For this review, take the finished solid that the model builds, in its own axes (mm). A direction names the side the tool comes from. Give positions to 0.01 mm unless a question says otherwise; leave off trailing zeros. Loops run counter-clockwise (first coordinate to the right, second up) from the corner with the lowest first, then second, coordinate; pieces in that order, holes last. Notation, with made-up numbers: M -38,-15.5 L -17,-15.5 A25 cw -17,16.5 Z; hole C 34.5,43.5 d9. An arc over 180 degrees is marked long. Use CSV: the item, a comma, the result in double quotes. Start each with the question number.
1. Insertion check: P1, Ø5, axis at x = 10.5, z = 10, coming from the +Y side; P2, Ø2.5, axis at x = 13.5, y = -1, coming from the +Z side; P3, Ø3, axis at x = 13.75, y = 0, coming from the -Z side; P4, Ø2, axis at x = -8, y = -4.5, coming from the +Z side. Each pin has a flat end and moves straight along its axis. Give the tip position at first contact, or say it passes through.
2. Take a section at B-B, the plane z = 18. Write out the cut boundary in (x, y).
3. To check wall thickness, follow line 1 (X direction, y = -8, z = 2); line 2 (X direction, y = 3.75, z = 16); line 3 (Z direction, x = 14.5, y = -3). State the ranges of each line that lie inside material, in increasing order. Write a range as [from, to].
4. The part is to be moulded in two halves that separate along X. For faces 5 (the face through (-3.75, 0, 11)), 6 (the face through (8.75, 0, 15)), 7 (the face through (-8.26, -9.49, 14.75)), say which applies: pulls with the +X half, pulls with the -X half, needs draft (parallel to the pull), parting line crosses it, or undercut.
5. Take a section at D-D, the plane x = 0. Write out the cut boundary in (y, z), and give its area (3 significant figures).
6. Take a section at C-C, the plane x = -13.75. Write out the cut boundary in (y, z), and give its area (3 significant figures).
7. Tool access review of faces 1 (the face through (8.26, 9.49, 14.5)), 2 (the face through (-4, -10, 12)), 3 (the face through (-11, -2, 5)), 4 (the face through (-8.26, 9.49, 14.75)): name each direction out of +Z, -Z, +X, -X, +Y, -Y from which nothing blocks a thin tool from reaching the whole face with its end or side.
8. Take a section at A-A, the plane y = 0. Write out the cut boundary in (x, z).
from build123d import *

# Parameters (mm, degrees)
F1_DEPTH      = 10
F1_DEPTH_BACK = 10
F2_R          = 2
F3_DEPTH      = 25
F4_SIZE       = 1


with BuildPart() as f1:
    # F0 (on Front) → F1 (new body, two sides)
    with BuildSketch(Plane.XZ) as f1_sk:
        with BuildLine():
            Line((3.75, 23.25), (3.75, 0))
            Line((3.75, 0), (18.75, 0))
            Line((18.75, 0), (18.75, 5))
            Line((18.75, 5), (8.75, 5))
            Line((8.75, 5), (8.75, 23.25))
            ThreePointArc((8.75, 23.25), (0, 32), (-8.75, 23.25))
            Line((-8.75, 23.25), (-8.75, 5))
            Line((-8.75, 5), (-18.75, 5))
            Line((-18.75, 5), (-18.75, 0))
            Line((-18.75, 0), (-3.75, 0))
            Line((-3.75, 0), (-3.75, 23.25))
            ThreePointArc((-3.75, 23.25), (0, 27), (3.75, 23.25))
        make_face()
    extrude(amount=-F1_DEPTH)
    extrude(f1_sk.sketch, amount=F1_DEPTH_BACK)

    # F2 (on face) → F3 (cut)
    with BuildSketch(Plane.XY.offset(5)):
        with Locations((-13.75, 0)):
            Circle(F2_R)
        with Locations((13.75, 0)):
            Circle(F2_R)
    extrude(amount=-F3_DEPTH, mode=Mode.SUBTRACT)

    # F4
    f4_edges = [f1.edges().sort_by_distance(p)[0] for p in [
        (11.75, 0, 5),
        (-15.75, 0, 5),
        (13.75, -10, 5),
        (18.75, 0, 5),
        (13.75, 10, 5),
        (8.75, 0, 5),
        (-8.75, 0, 5),
        (-13.75, 10, 5),
        (-13.75, -10, 5),
        (-18.75, 0, 5),
        (8.75, 10, 14.125),
        (0, 10, 32),
        (-8.75, 10, 14.125),
        (8.75, -10, 14.125),
        (0, -10, 32),
        (-8.75, -10, 14.125),
    ]]
    chamfer(f4_edges, length=F4_SIZE)


solid = f1.part
Result set:
1,P1,"y = 9.75"
1,P2,"z = 4.28"
1,P3,"through"
1,P4,"z = 28.5"
2,outline,"M -8.75,-9 L -7.75,-10 L -3.75,-10 L -3.75,10 L -7.75,10 L -8.75,9 Z; M 3.75,-10 L 7.75,-10 L 8.75,-9 L 8.75,9 L 7.75,10 L 3.75,10 Z"
3,line 1,"[-18.75, -3.75], [3.75, 18.75]"
3,line 2,"[-8.75, -3.75], [3.75, 8.75]"
3,line 3,"[0, 5]"
4,face 5,"undercut"
4,face 6,"pulls with the +X half"
4,face 7,"pulls with the -X half"
5,outline,"M -10,27 L 10,27 L 10,31 L 9,32 L -9,32 L -10,31 Z"
5,area,"99.0 mm2"
6,outline,"M -10,0 L -2,0 L -2,4 L -3,5 L -9,5 L -10,4 Z; M 2,0 L 10,0 L 10,4 L 9,5 L 3,5 L 2,4 Z"
6,area,"78.0 mm2"
7,face 1,"+Z, +X, +Y"
7,face 2,"+Z, -Z, +X, -X, -Y"
7,face 3,"+Z, -X, +Y, -Y"
7,face 4,"+Z, -X, +Y"
8,outline,"M -18.75,0 L -15.75,0 L -15.75,4 L -16.75,5 L -17.75,5 L -18.75,4 Z; M -11.75,0 L -3.75,0 L -3.75,23.25 A3.75 cw 3.75,23.25 L 3.75,0 L 11.75,0 L 11.75,4 L 10.75,5 L 9.75,5 L 8.75,6 L 8.75,23.25 A8.75 ccw -8.75,23.25 L -8.75,6 L -9.75,5 L -10.75,5 L -11.75,4 Z; M 15.75,0 L 18.75,0 L 18.75,4 L 17.75,5 L 16.75,5 L 15.75,4 Z"
